Source: CAD feature listing. Evaluate the final solid. Frame: model axes, mm. A direction names the side the tool comes from. Give positions to 0.01 mm unless a question says otherwise; leave off trailing zeros. Write each loop counter-clockwise with the first axis right and the second up, starting at its lowest first coordinate (ties: lowest second). Pieces come first, ordered by that corner, then holes.
Autodesk Inventor part; units mm, degrees
ref_plane "YZ Plane" through (0, 0, 0) normal (1, 0, 0) x (0, 1, 0)
ref_plane "XZ Plane" through (0, 0, 0) normal (0, 1, 0) x (-1, 0, 0)
ref_plane "XY Plane" through (0, 0, 0) normal (0, 0, 1) x (1, 0, 0)
sketch "Sketch1" plane through (0, 0, 0) normal (0, 0, 1) x (1, 0, 0)
  line L0 (0, 0) -> (0, 20.872) construction
  line L1 (0, 0) -> (7.1878, 0) construction
  line L2 (0, 6.45) -> (0.3969, 6.45)
  line L3 (0.3969, 6.45) -> (0.71, 4.674) construction
  line L4 (0.5535, 5.562) -> (2.6468, 5.9311) construction
  arc A0 (0.71, 4.674) -> (0.3969, 6.45) centre (-1.785, 5.1496) ccw
  line L5 (0, 6.45) -> (-0.3969, 6.45)
  arc A1 (-0.3969, 6.45) -> (-0.71, 4.674) centre (1.785, 5.1496) ccw
  line L6 (-0.3969, 6.45) -> (0.3969, 6.45)
  line L7 (-0.3969, 6.45) -> (0.3969, 6.45)
  line L8 (-3.225, 5.5858) -> (-2.8813, 5.7843)
  arc A2 (-1.7221, 4.4028) -> (-2.8813, 5.7843) centre (-4.1207, 3.5672) ccw
  arc A3 (-3.5687, 5.3874) -> (-2.9519, 3.6928) centre (-1.0289, 5.3522) ccw
  line L9 (-3.225, 5.5858) -> (-3.5687, 5.3874)
  line L10 (-5.5858, 3.225) -> (-5.3874, 3.5687)
  arc A4 (-3.6928, 2.9519) -> (-5.3874, 3.5687) centre (-5.3522, 1.0289) ccw
  arc A5 (-5.7843, 2.8813) -> (-4.4028, 1.7221) centre (-3.5672, 4.1207) ccw
  line L11 (-5.5858, 3.225) -> (-5.7843, 2.8813)
  line L12 (-6.45, 0) -> (-6.45, 0.3969)
  arc A6 (-4.674, 0.71) -> (-6.45, 0.3969) centre (-5.1496, -1.785) ccw
  arc A7 (-6.45, -0.3969) -> (-4.674, -0.71) centre (-5.1496, 1.785) ccw
  line L13 (-6.45, 0) -> (-6.45, -0.3969)
  line L14 (-5.5858, -3.225) -> (-5.7843, -2.8813)
  arc A8 (-4.4028, -1.7221) -> (-5.7843, -2.8813) centre (-3.5672, -4.1207) ccw
  arc A9 (-5.3874, -3.5687) -> (-3.6928, -2.9519) centre (-5.3522, -1.0289) ccw
  line L15 (-5.5858, -3.225) -> (-5.3874, -3.5687)
  line L16 (-3.225, -5.5858) -> (-3.5687, -5.3874)
  arc A10 (-2.9519, -3.6928) -> (-3.5687, -5.3874) centre (-1.0289, -5.3522) ccw
  arc A11 (-2.8813, -5.7843) -> (-1.7221, -4.4028) centre (-4.1207, -3.5672) ccw
  line L17 (-3.225, -5.5858) -> (-2.8813, -5.7843)
  line L18 (0, -6.45) -> (-0.3969, -6.45)
  arc A12 (-0.71, -4.674) -> (-0.3969, -6.45) centre (1.785, -5.1496) ccw
  arc A13 (0.3969, -6.45) -> (0.71, -4.674) centre (-1.785, -5.1496) ccw
  line L19 (0, -6.45) -> (0.3969, -6.45)
  line L20 (3.225, -5.5858) -> (2.8813, -5.7843)
  arc A14 (1.7221, -4.4028) -> (2.8813, -5.7843) centre (4.1207, -3.5672) ccw
  arc A15 (3.5687, -5.3874) -> (2.9519, -3.6928) centre (1.0289, -5.3522) ccw
  line L21 (3.225, -5.5858) -> (3.5687, -5.3874)
  line L22 (5.5858, -3.225) -> (5.3874, -3.5687)
  arc A16 (3.6928, -2.9519) -> (5.3874, -3.5687) centre (5.3522, -1.0289) ccw
  arc A17 (5.7843, -2.8813) -> (4.4028, -1.7221) centre (3.5672, -4.1207) ccw
  line L23 (5.5858, -3.225) -> (5.7843, -2.8813)
  line L24 (6.45, 0) -> (6.45, -0.3969)
  arc A18 (4.674, -0.71) -> (6.45, -0.3969) centre (5.1496, 1.785) ccw
  arc A19 (6.45, 0.3969) -> (4.674, 0.71) centre (5.1496, -1.785) ccw
  line L25 (6.45, 0) -> (6.45, 0.3969)
  line L26 (5.5858, 3.225) -> (5.7843, 2.8813)
  arc A20 (4.4028, 1.7221) -> (5.7843, 2.8813) centre (3.5672, 4.1207) ccw
  arc A21 (5.3874, 3.5687) -> (3.6928, 2.9519) centre (5.3522, 1.0289) ccw
  line L27 (5.5858, 3.225) -> (5.3874, 3.5687)
  line L28 (3.225, 5.5858) -> (3.5687, 5.3874)
  arc A22 (2.9519, 3.6928) -> (3.5687, 5.3874) centre (1.0289, 5.3522) ccw
  arc A23 (2.8813, 5.7843) -> (1.7221, 4.4028) centre (4.1207, 3.5672) ccw
  line L29 (3.225, 5.5858) -> (2.8813, 5.7843)
  line L30 (-1.7221, 4.4028) -> (-0.71, 4.674) construction
  arc A24 (1.7221, 4.4028) -> (0.71, 4.674) centre (0, 0) ccw
  arc A25 (3.6928, 2.9519) -> (2.9519, 3.6928) centre (0, 0) ccw
  arc A26 (4.674, 0.71) -> (4.4028, 1.7221) centre (0, 0) ccw
  arc A27 (4.4028, -1.7221) -> (4.674, -0.71) centre (0, 0) ccw
  arc A28 (2.9519, -3.6928) -> (3.6928, -2.9519) centre (0, 0) ccw
  arc A29 (0.71, -4.674) -> (1.7221, -4.4028) centre (0, 0) ccw
  arc A30 (-1.7221, -4.4028) -> (-0.71, -4.674) centre (0, 0) ccw
  arc A31 (-3.6928, -2.9519) -> (-2.9519, -3.6928) centre (0, 0) ccw
  arc A32 (-4.674, -0.71) -> (-4.4028, -1.7221) centre (0, 0) ccw
  arc A33 (-4.4028, 1.7221) -> (-4.674, 0.71) centre (0, 0) ccw
  arc A34 (-0.71, 4.674) -> (-1.7221, 4.4028) centre (0, 0) ccw
  arc A35 (-2.9519, 3.6928) -> (-3.6928, 2.9519) centre (0, 0) ccw
  dimension "d0" = 0.7937
  dimension "d4" = 360
  dimension "d6" = 80
  dimension "d7" = 1.8034
  dimension "d8" = 2.54
  dimension "d11" = 1.0477
extrude "Extrusion1" add sketch "Sketch1" along normal blind 1.5875
sketch "Sketch2" plane through (0, 0, 1.5875) normal (0, 0, 1) x (1, 0, 0)
  arc A0 (1.7221, 4.4028) -> (0.71, 4.674) centre (0, 0) ccw
  circle A1 centre (0, 0) radius 1.5875
  dimension "d12" = 3.175
extrude "Extrusion2" cut sketch "Sketch2" against normal blind 1.5875
sketch "Sketch3" plane through (0, 0, 1.5875) normal (0, 0, 1) x (1, 0, 0)
  circle A0 centre (0, 0) radius 1.5875
  arc A1 (-0.3969, 6.45) -> (-0.71, 4.674) centre (1.785, 5.1496) ccw
  arc A2 (-0.71, 4.674) -> (-1.7221, 4.4028) centre (0, 0) ccw
  arc A3 (-1.7221, 4.4028) -> (-2.8813, 5.7843) centre (-4.1207, 3.5672) ccw
  line L0 (-2.8813, 5.7843) -> (-3.5687, 5.3874)
  arc A4 (-3.5687, 5.3874) -> (-2.9519, 3.6928) centre (-1.0289, 5.3522) ccw
  arc A5 (-2.9519, 3.6928) -> (-3.6928, 2.9519) centre (0, 0) ccw
  arc A6 (-3.6928, 2.9519) -> (-5.3874, 3.5687) centre (-5.3522, 1.0289) ccw
  line L1 (-5.3874, 3.5687) -> (-5.7843, 2.8813)
  arc A7 (-5.7843, 2.8813) -> (-4.4028, 1.7221) centre (-3.5672, 4.1207) ccw
  arc A8 (-4.4028, 1.7221) -> (-4.674, 0.71) centre (0, 0) ccw
  arc A9 (-4.674, 0.71) -> (-6.45, 0.3969) centre (-5.1496, -1.785) ccw
  line L2 (-6.45, 0.3969) -> (-6.45, -0.3969)
  arc A10 (-6.45, -0.3969) -> (-4.674, -0.71) centre (-5.1496, 1.785) ccw
  arc A11 (-4.674, -0.71) -> (-4.4028, -1.7221) centre (0, 0) ccw
  arc A12 (-4.4028, -1.7221) -> (-5.7843, -2.8813) centre (-3.5672, -4.1207) ccw
  line L3 (-5.7843, -2.8813) -> (-5.3874, -3.5687)
  arc A13 (-5.3874, -3.5687) -> (-3.6928, -2.9519) centre (-5.3522, -1.0289) ccw
  arc A14 (-3.6928, -2.9519) -> (-2.9519, -3.6928) centre (0, 0) ccw
  arc A15 (-2.9519, -3.6928) -> (-3.5687, -5.3874) centre (-1.0289, -5.3522) ccw
  line L4 (-3.5687, -5.3874) -> (-2.8813, -5.7843)
  arc A16 (-2.8813, -5.7843) -> (-1.7221, -4.4028) centre (-4.1207, -3.5672) ccw
  arc A17 (-1.7221, -4.4028) -> (-0.71, -4.674) centre (0, 0) ccw
  arc A18 (-0.71, -4.674) -> (-0.3969, -6.45) centre (1.785, -5.1496) ccw
  line L5 (-0.3969, -6.45) -> (0.3969, -6.45)
  arc A19 (0.3969, -6.45) -> (0.71, -4.674) centre (-1.785, -5.1496) ccw
  arc A20 (0.71, -4.674) -> (1.7221, -4.4028) centre (0, 0) ccw
  arc A21 (1.7221, -4.4028) -> (2.8813, -5.7843) centre (4.1207, -3.5672) ccw
  line L6 (2.8813, -5.7843) -> (3.5687, -5.3874)
  arc A22 (3.5687, -5.3874) -> (2.9519, -3.6928) centre (1.0289, -5.3522) ccw
  arc A23 (2.9519, -3.6928) -> (3.6928, -2.9519) centre (0, 0) ccw
  arc A24 (3.6928, -2.9519) -> (5.3874, -3.5687) centre (5.3522, -1.0289) ccw
  line L7 (5.3874, -3.5687) -> (5.7843, -2.8813)
  arc A25 (5.7843, -2.8813) -> (4.4028, -1.7221) centre (3.5672, -4.1207) ccw
  arc A26 (4.4028, -1.7221) -> (4.674, -0.71) centre (0, 0) ccw
  arc A27 (4.674, -0.71) -> (6.45, -0.3969) centre (5.1496, 1.785) ccw
  line L8 (6.45, -0.3969) -> (6.45, 0.3969)
  arc A28 (6.45, 0.3969) -> (4.674, 0.71) centre (5.1496, -1.785) ccw
  arc A29 (4.674, 0.71) -> (4.4028, 1.7221) centre (0, 0) ccw
  arc A30 (4.4028, 1.7221) -> (5.7843, 2.8813) centre (3.5672, 4.1207) ccw
  line L9 (5.7843, 2.8813) -> (5.3874, 3.5687)
  arc A31 (5.3874, 3.5687) -> (3.6928, 2.9519) centre (5.3522, 1.0289) ccw
  arc A32 (3.6928, 2.9519) -> (2.9519, 3.6928) centre (0, 0) ccw
  arc A33 (2.9519, 3.6928) -> (3.5687, 5.3874) centre (1.0289, 5.3522) ccw
  line L10 (3.5687, 5.3874) -> (2.8813, 5.7843)
  arc A34 (2.8813, 5.7843) -> (1.7221, 4.4028) centre (4.1207, 3.5672) ccw
  arc A35 (1.7221, 4.4028) -> (0.71, 4.674) centre (0, 0) ccw
  arc A36 (0.71, 4.674) -> (0.3969, 6.45) centre (-1.785, 5.1496) ccw
  line L11 (0.3969, 6.45) -> (-0.3969, 6.45)
  line L12 (-0.71, 4.674) -> (0.71, 4.674)
  arc A37 (0.71, 4.674) -> (0.3969, 6.45) centre (-1.785, 5.1496) ccw
  line L13 (0.3969, 6.45) -> (-0.3969, 6.45)
  arc A38 (-0.3969, 6.45) -> (-0.71, 4.674) centre (1.785, 5.1496) ccw
properties part number "Sun"
1. Access query for faces 5 (the cylindrical face through (-2.183, 5.21, 0.783)), 6 (the cylindrical face through (5.19, -2.167, 0.783)), 7 (the cylindrical face through (-2.167, -5.19, 0.783)), 8 (the cylindrical face through (-5.603, 0.714, 0.783)). Directions: +Z, -Z, +X, -X, +Y, -Y. A direction counts if a zero-diameter tool reaches every point of the face in a straight line with its end or side. Return the directions, or none.
2. Line query: probe 1 along Y at (x, z) = (0, 1.35); probe 2 along Y at (x, z) = (5.5, 0.7). Output: solid intervals per line, ascending.
3. Pull-direction query (Y, two-part tool) for faces 1 (the cylindrical face through (-4.5, 3.42, 0.78)), 2 (the cylindrical face through (3.41, -4.47, 0.78)), 3 (the flat face through (1.3, -1.3, 0)), 4 (the cylindrical face through (2.183, -5.21, 0.783)); classes: pulls with the +Y half, pulls with the -Y half, needs draft (parallel to the pull), parting line crosses it, or undercut.
4. Section query A-A (x = 0). Return loops of the section in (y, z).
5. Pin query (flat end, axial travel): P1, Ø2.5, axis at x = 0, y = 0, coming from the -Z side. Return the tip coordinate at first contact, or that it passes through.
The answers:
1. face 5: +Z, -Z, +Y
1. face 6: +Z, -Z, +X
1. face 7: +Z, -Z, -Y
1. face 8: +Z, -Z
2. probe 1: y = -6.45 to -1.59, 1.59 to 6.45
2. probe 2: y = -3.37 to -2.47, -0.73 to 0.73, 2.47 to 3.37
3. face 1: pulls with the +Y half
3. face 2: undercut
3. face 3: needs draft
3. face 4: pulls with the -Y half
4. outline: (-6.45, 0) - (-1.59, 0) - (-1.59, 1.59) - (-6.45, 1.59) - close; (1.59, 0) - (6.45, 0) - (6.45, 1.59) - (1.59, 1.59) - close
5. P1: passes through
